Model file for the job. Use its own axes, mm. Coordinates: 2 decimals unless noted, no trailing zeros. Use CSV: the item, a comma, the result in double quotes. Start each with the question number.
(1) Probe L1, parallel to X at y = -6.95, z = 260; L2, parallel to Y at x = -5, z = 224; L3, parallel to Y at x = 2.5, z = 159. List the from-to ranges inside material, lowest first.
(2) Pin check, flat tips, straight feed: pin 1 Ø3 at (x, z) = (0, 85) entering from +Y; pin 2 Ø5.5 at (x, z) = (0, 35) entering from +Y; pin 3 Ø7 at (x, z) = (0, 85) entering from +Y. Stop position of each tip, or through.
(3) Cut at A-A on y = -6.25. Give the number of separate pieces and of enclosed holes in the cut face, plus the area to 3 significant figures.
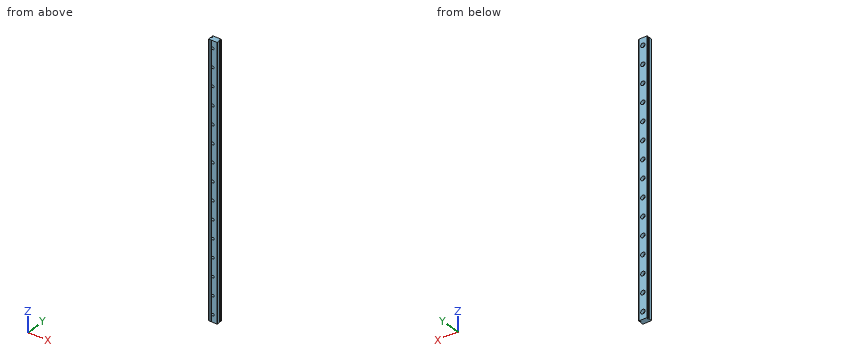
```python
from build123d import *

# Parameters (mm, degrees)
BOSS_EXTRUDE1_DEPTH = 370
SKETCH2_R           = 1.75
CUT_EXTRUDE1_DEPTH  = 8.999998
SKETCH2_3_R         = 3
CUT_EXTRUDE2_DEPTH  = 4.5


with BuildPart() as part:
    # Sketch1 → Boss-Extrude1 (new body)
    with BuildSketch(Plane.XY):
        with BuildLine():
            Line((5.5, -7.999998), (6, -7.499998))
            Line((6, -7.499998), (6, -3.85787958))
            ThreePointArc((6, -3.85787958), (5.9576137, -3.718608076), (5.844827586, -3.626562203))
            ThreePointArc((5.844827586, -3.626562203), (5.51524529, -3.424071402), (5.267205011, -3.12724985))
            ThreePointArc((5.267205011, -3.12724985), (5.185241933, -3.042985123), (5.073828324, -3.005495145))
            Line((5.073828324, -3.005495145), (4.728211064, -2.975257553))
            ThreePointArc((4.728211064, -2.975257553), (4.565680666, -2.89510643), (4.5, -2.726208878))
            Line((4.5, -2.726208878), (4.5, -2.273787121))
            ThreePointArc((4.5, -2.273787121), (4.565680666, -2.10488957), (4.728211064, -2.024738447))
            Line((4.728211064, -2.024738447), (5.09477657, -1.992668121))
            ThreePointArc((5.09477657, -1.992668121), (5.203244499, -1.957004425), (5.284541491, -1.876829678))
            ThreePointArc((5.284541491, -1.876829678), (5.527906161, -1.597614221), (5.844827586, -1.405915383))
            ThreePointArc((5.844827586, -1.405915383), (5.9576137, -1.31386951), (6, -1.174598006))
            Line((6, -1.174598006), (6, -0.5))
            Line((6, -0.5), (5.5, 0))
            Line((5.5, 0), (-5.5, 0))
            Line((-5.5, 0), (-6, -0.5))
            Line((-6, -0.5), (-6, -1.174598006))
            ThreePointArc((-6, -1.174598006), (-5.9576137, -1.31386951), (-5.844827586, -1.405915383))
            ThreePointArc((-5.844827586, -1.405915383), (-5.527906161, -1.597614221), (-5.284541491, -1.876829678))
            ThreePointArc((-5.284541491, -1.876829678), (-5.203244499, -1.957004425), (-5.09477657, -1.992668121))
            Line((-5.09477657, -1.992668121), (-4.728211064, -2.024738447))
            ThreePointArc((-4.728211064, -2.024738447), (-4.565680666, -2.10488957), (-4.5, -2.273787121))
            Line((-4.5, -2.273787121), (-4.5, -2.726208878))
            ThreePointArc((-4.5, -2.726208878), (-4.565680666, -2.89510643), (-4.728211064, -2.975257553))
            Line((-4.728211064, -2.975257553), (-5.073828324, -3.005495145))
            ThreePointArc((-5.073828324, -3.005495145), (-5.185241932, -3.042985123), (-5.267205011, -3.12724985))
            ThreePointArc((-5.267205011, -3.12724985), (-5.51524529, -3.424071402), (-5.844827586, -3.626562203))
            ThreePointArc((-5.844827586, -3.626562203), (-5.9576137, -3.718608076), (-6, -3.85787958))
            Line((-6, -3.85787958), (-6, -7.499998))
            Line((-6, -7.499998), (-5.5, -7.999998))
            Line((-5.5, -7.999998), (-2.4, -7.999998))
            ThreePointArc((-2.4, -7.999998), (-2, -7.799998), (-1.6, -7.999998))
            Line((-1.6, -7.999998), (5.5, -7.999998))
        make_face()
    extrude(amount=BOSS_EXTRUDE1_DEPTH)

    # Sketch2 → Cut-Extrude1 (cut, through all)
    with BuildSketch(Plane(origin=(0, 0, 0), x_dir=(1, 0, 0), z_dir=(0, 1, 0))):
        with Locations((0, -10)):
            Circle(SKETCH2_R)
        with Locations((0, -35)):
            Circle(SKETCH2_R)
        with Locations((0, -60)):
            Circle(SKETCH2_R)
        with Locations((0, -85)):
            Circle(SKETCH2_R)
        with Locations((0, -110)):
            Circle(SKETCH2_R)
        with Locations((0, -135)):
            Circle(SKETCH2_R)
        with Locations((0, -160)):
            Circle(SKETCH2_R)
        with Locations((0, -185)):
            Circle(SKETCH2_R)
        with Locations((0, -210)):
            Circle(SKETCH2_R)
        with Locations((0, -235)):
            Circle(SKETCH2_R)
        with Locations((0, -260)):
            Circle(SKETCH2_R)
        with Locations((0, -285)):
            Circle(SKETCH2_R)
        with Locations((0, -310)):
            Circle(SKETCH2_R)
        with Locations((0, -335)):
            Circle(SKETCH2_R)
        with Locations((0, -360)):
            Circle(SKETCH2_R)
        with Locations((0, -385)):
            Circle(SKETCH2_R)
        with Locations((0, -410)):
            Circle(SKETCH2_R)
    extrude(amount=-CUT_EXTRUDE1_DEPTH, mode=Mode.SUBTRACT)

    # Sketch2<3> → Cut-Extrude2 (cut)
    with BuildSketch(Plane(origin=(0, 0, 0), x_dir=(1, 0, 0), z_dir=(0, 1, 0))):
        with Locations((0, -10)):
            Circle(SKETCH2_3_R)
        with Locations((0, -35)):
            Circle(SKETCH2_3_R)
        with Locations((0, -60)):
            Circle(SKETCH2_3_R)
        with Locations((0, -85)):
            Circle(SKETCH2_3_R)
        with Locations((0, -110)):
            Circle(SKETCH2_3_R)
        with Locations((0, -135)):
            Circle(SKETCH2_3_R)
        with Locations((0, -160)):
            Circle(SKETCH2_3_R)
        with Locations((0, -185)):
            Circle(SKETCH2_3_R)
        with Locations((0, -210)):
            Circle(SKETCH2_3_R)
        with Locations((0, -235)):
            Circle(SKETCH2_3_R)
        with Locations((0, -260)):
            Circle(SKETCH2_3_R)
        with Locations((0, -285)):
            Circle(SKETCH2_3_R)
        with Locations((0, -310)):
            Circle(SKETCH2_3_R)
        with Locations((0, -335)):
            Circle(SKETCH2_3_R)
        with Locations((0, -360)):
            Circle(SKETCH2_3_R)
        with Locations((0, -385)):
            Circle(SKETCH2_3_R)
        with Locations((0, -410)):
            Circle(SKETCH2_3_R)
    extrude(amount=-CUT_EXTRUDE2_DEPTH, mode=Mode.SUBTRACT)


solid = part.part
```
Outcome:
1,L1,"-6 to -1.75, 1.75 to 6"
1,L2,"-8 to -3, -2 to 0"
1,L3,"-8 to -4.5"
2,pin 1,"through"
2,pin 2,"y = -4.5"
2,pin 3,"y = 0"
3,separate pieces,"1"
3,enclosed holes,"15"
3,area,"4,300 mm2"
